Answer from the drawing. Dimensions are ordinates in mm from the lowest x, y and z of the part. Give positions to 0.01 mm unless a question says otherwise; leave off trailing zeros. Order: outer loops, then holes, each group sorted by start corner. A loop starts at its lowest first (then second) coordinate and runs counter-clockwise, first axis right, second up. Notation, with made-up numbers: M 19,22.5 L 66,22.5 A8 ccw 66,27.5 Z; hole C 84.25,77.25 d11. An arc over 180 degrees is marked long. One line per item, written item: value.
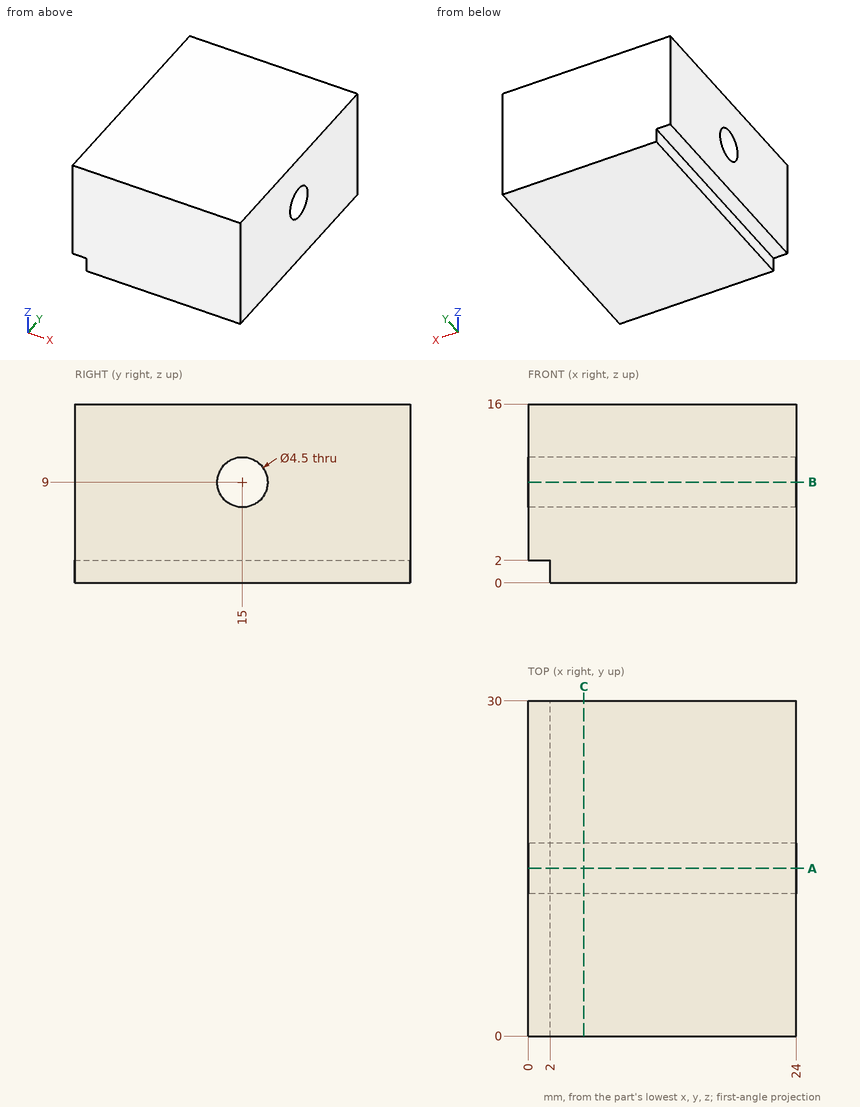
(1) Section C-C, the plane x = 5 is taken. Give the vertices of the cut face in (y, z).
Findings:
outline: M 0,0 L 30,0 L 30,16 L 0,16 Z; hole C 15,9 d4.5
(2) Find the intervals of material crossed by probe 1 along Y at (x, z) = (14.25, 9); probe 2 along Y at (x, z) = (23, 10.25); probe 3 along X at (y, z) = (10.75, 1.75), in increasing order. Write a range as from..to.
Findings:
probe 1: y = 0..12.75, 17.25..30
probe 2: y = 0..13.13, 16.87..30
probe 3: x = 2..24
(3) Section B-B, the plane z = 9 is taken. Give the vertices of the cut face in (x, y), then the cut area to 3 significant figures.
Findings:
outline: M 0,0 L 24,0 L 24,12.75 L 0,12.75 Z; M 0,17.25 L 24,17.25 L 24,30 L 0,30 Z
area: 612 mm^2
(4) Section A-A, the plane y = 15 is taken. Give the vertices of the cut face in (x, z), then the cut area to 3 significant figures.
Findings:
outline: M 0,2 L 2,2 L 2,0 L 24,0 L 24,6.75 L 0,6.75 Z; M 0,11.25 L 24,11.25 L 24,16 L 0,16 Z
area: 272 mm^2
(5) Given P1, Ø0.6, axis at y = 7.5, z = 0.5, coming from the -X side; P2, Ø4, axis at y = 15, z = 9, coming from the -X side; P3, Ø1.6, axis at x = 0.5, y = 12, coming from the -Z side, each flat-ended and moving along its own axis, determine where each tip first touches the part or whether it passes through.
Findings:
P1: stops at x = 2
P2: passes through
P3: stops at z = 2
